Model file for the job. Use its own axes, mm. A direction names the side the tool comes from. Round coordinates to 2 decimals unless told otherwise and drop trailing zeros. Order: outer loops, then holes, each group sorted by start corner. A loop starts at its lowest first (then second) coordinate and runs counter-clockwise, first axis right, second up. Notation, with made-up numbers: (64.5, 28) -> (71.5, 28) arc R12 ccw to (71.5, 32) -> close; hole circle Ø10 at (72.25, 58). An arc over 180 degrees is marked (long way). Use CSV: the item, a comma, the result in double quotes.
```python
from build123d import *

# Parameters (mm, degrees)
MODEL_R                     = 12.1
EXTRUDE_318_DEPTH           = 0.5
CUT_EXTRUDE_1_DEPTH         = 18.141178489
EXTRUDE_892_DEPTH           = 1
PATTERN_CIRCULAR_946_COUNT  = 19
HOLE_WIZARD_M1_6_AT_2_COUNT = 2
HOLE_WIZARD_M1_6_AT_2_PITCH = 8.660254038
HOLE_WIZARD_M1_6_AT_3_COUNT = 2
HOLE_WIZARD_M1_6_AT_3_PITCH = 8.660254038


with BuildPart() as part:
    # Model → Extrude 318 (new, symmetric)
    with BuildSketch(Plane.XY):
        Circle(MODEL_R)
    extrude(amount=EXTRUDE_318_DEPTH, both=True)

    # Эскиз3 → Вырез-Вытянуть1 (cut, through all)
    with BuildSketch(Plane.XY.offset(0.5)):
        with BuildLine():
            Line((2, -1.5), (-2, -1.5))
            ThreePointArc((-2, -1.5), (-2.5, 0), (-2, 1.5))
            Line((-2, 1.5), (2, 1.5))
            ThreePointArc((2, 1.5), (2.5, 0), (2, -1.5))
        make_face()
    extrude(amount=-CUT_EXTRUDE_1_DEPTH, mode=Mode.SUBTRACT)

    # Эскиз4 → Extrude 892 (add)
    with BuildSketch(Plane.XY.offset(0.5)):
        with BuildLine():
            Line((-0.5, 11.6), (0.5, 11.6))
            Line((0.5, 11.6), (0.29607573, 12.848364887))
            ThreePointArc((0.29607573, 12.848364887), (0, 13.1), (-0.29607573, 12.848364887))
            Line((-0.29607573, 12.848364887), (-0.5, 11.6))
        make_face()
    extrude_892 = extrude(amount=-EXTRUDE_892_DEPTH)

    # Pattern Circular 946: Extrude 892 ×19 about axis
    pattern_circular_946_axis = Axis((0, 0, 0), (0, 0, 1))
    for i in range(1, PATTERN_CIRCULAR_946_COUNT):
        add(extrude_892.rotate(pattern_circular_946_axis, i * 360 / PATTERN_CIRCULAR_946_COUNT))

    # Эскиз6 → Крепление шестерни M1.6 (revolve, cut)
    with BuildSketch(Plane(origin=(4.330127019, 2.5, -0.5), x_dir=(0, 1, 0), z_dir=(1, 0, 0))):
        Polygon((0, 0), (0, 1), (0.9, 1), (0.9, 0.9), (1.8, 0), align=None)
    hole_wizard_m1_6 = revolve(axis=Axis((4.330127019, 2.5, -6.85), (0, 0, 1)), mode=Mode.SUBTRACT)

    # Крепление шестерни M1.6 at 2: Крепление шестерни M1.6 ×2
    with Locations(*[Vector(-0.49999999999999795, -0.8660254037844399, 0) * (i * HOLE_WIZARD_M1_6_AT_2_PITCH) for i in range(1, HOLE_WIZARD_M1_6_AT_2_COUNT)]):
        add(hole_wizard_m1_6, mode=Mode.SUBTRACT)

    # Крепление шестерни M1.6 at 3: Крепление шестерни M1.6 ×2
    with Locations(*[(-i * HOLE_WIZARD_M1_6_AT_3_PITCH, 0, 0) for i in range(1, HOLE_WIZARD_M1_6_AT_3_COUNT)]):
        add(hole_wizard_m1_6, mode=Mode.SUBTRACT)


solid = part.part
```
Q1. Cut at A-A (x = 0). Give the cut face in (y, z), plus the area to 3 significant figures.
From the geometry:
outline,"(-12.1, -0.5) -> (-6.8, -0.5) -> (-5.9, 0.4) -> (-5.9, 0.5) -> (-12.1, 0.5) -> close; (-4.1, 0.4) -> (-3.2, -0.5) -> (-1.5, -0.5) -> (-1.5, 0.5) -> (-4.1, 0.5) -> close; (1.5, -0.5) -> (13.1, -0.5) -> (13.1, 0.5) -> (1.5, 0.5) -> close"
area,"19.6 mm²"
Q2. Which spindle directions (+Z, -Z, +X, -X, +Y, -Y) get a long thin tool onto all of the face, cutting with end or side? Do faces 4 (the cylindrical face through (3.91, -11.45, 0.01)), 5 (the flat face through (0, -1.5, 0)), 6 (the cylindrical face through (-12.057, 1.021, 0.007)), 7 (the cylindrical face through (11.724, -2.992, 0.007)). Say none if no direction does.
From the geometry:
face 4,"+Z, -Z, -Y"
face 5,"+Z, -Z"
face 6,"+Z, -Z, -X"
face 7,"+Z, -Z, +X"
Q3. Probe line 1 along X through (y, z) = (3.5, 0); line 2 along X through (y, z) = (0, 0.3); line 3 along X through (y, z) = (-1, 0.3). List the from-to ranges inside material, lowest first.
From the geometry:
line 1,"x = -11.58 to -5.16, -3.5 to 3.5, 5.16 to 11.58"
line 2,"x = -12.1 to -2.5, 2.5 to 12.1"
line 3,"x = -13.05 to -2.29, 2.29 to 13.05"
Q4. Cut at B-B (z = -0.25). State how many separate pieces and enclosed holes the cut face has, plus the area to 3 significant figures.
From the geometry:
separate pieces,"1"
enclosed holes,"4"
area,"436 mm²"
Q5. Mould opens along X. For faces 1 (the cylindrical face through (12.06, 0.98, 0.01)), 2 (the cylindrical face through (-3.95, -11.437, 0.007)), 3 (the cylindrical face through (-11.735, -2.949, 0.007)) say: +X half, -X half, draft (parallel to the pull), parting line (faces both ways), or undercut.
From the geometry:
face 1,"+X half"
face 2,"undercut"
face 3,"-X half"
Q6. Pin check, flat tip, straight feed: pin 1 (2 mm diameter, centred on x = 0, y = -5, fed in from -Z). Stop position of the tip, or through.
From the geometry:
pin 1,"stops at z = 0.3"
Q7. Cut at C-C (y = 7.75). Give the cut face in (x, z).
From the geometry:
outline,"(-9.29, -0.5) -> (9.29, -0.5) -> (9.29, 0.5) -> (-9.29, 0.5) -> close"
